from build123d import *

# Parameters (mm, degrees)
SKETCH1_R           = 5.5
SKETCH1_R_2         = 1.5
SKETCH1_R_3         = 4.5
BOSS_EXTRUDE1_DEPTH = 5
SKETCH4_R           = 6.1
CUT_EXTRUDE1_DEPTH  = 3.5
SKETCH5_R           = 1.5
CUT_EXTRUDE2_DEPTH  = 5
SKETCH6_R           = 1.5
CUT_EXTRUDE3_DEPTH  = 10
SKETCH7_R           = 2.9
CUT_EXTRUDE4_DEPTH  = 3.3


with BuildPart() as part:
    # Sketch1 → Boss-Extrude1 (new body)
    with BuildSketch(Plane.XY):
        with BuildLine():
            Line((-58.308676511, 22.996128985), (58.308676511, 22.996128985))
            Line((58.308676511, 22.996128985), (75.629184587, 15))
            Line((75.629184587, 15), (90.85122644, 7.972642053))
            ThreePointArc((90.85122644, 7.972642053), (87.163327852, -21.339018917), (58.308676511, -15))
            Line((58.308676511, -15), (7, -15))
            Line((7, -15), (2.757359313, -19.242640687))
            ThreePointArc((2.757359313, -19.242640687), (0, -20.384776311), (-2.757359313, -19.242640687))
            Line((-2.757359313, -19.242640687), (-7, -15))
            Line((-7, -15), (-58.308676511, -15))
            ThreePointArc((-58.308676511, -15), (-73.76298075, -27.603590324), (-89.217284989, -15))
            ThreePointArc((-89.217284989, -15), (-87.141316573, 1.955509585), (-75.243665272, 14.212949924))
            Line((-75.243665272, 14.212949924), (-58.308676511, 22.996128985))
        make_face()
        with Locations((-74.370815413, -15)):
            Circle(SKETCH1_R, mode=Mode.SUBTRACT)
        with Locations(Location((-74.370815413, -7, 0), (0, 0, 180))):
            Circle(SKETCH1_R_2, mode=Mode.SUBTRACT)
        with Locations((75.629184587, -15)):
            Circle(SKETCH1_R_3, mode=Mode.SUBTRACT)
        with Locations((0, -15.003871015)):
            Circle(SKETCH1_R_2, mode=Mode.SUBTRACT)
        with Locations(Location((-66.370815413, -15, 0), (0, 0, 180))):
            Circle(SKETCH1_R_2, mode=Mode.SUBTRACT)
        with Locations(Location((-74.370815413, -23, 0), (0, 0, 180))):
            Circle(SKETCH1_R_2, mode=Mode.SUBTRACT)
        with Locations(Location((-82.370815413, -15, 0), (0, 0, 180))):
            Circle(SKETCH1_R_2, mode=Mode.SUBTRACT)
        with BuildLine():
            Line((-58.308676511, -4.003871015), (58.308676511, -4.003871015))
            ThreePointArc((58.308676511, -4.003871015), (61.808676511, -0.503871015), (58.308676511, 2.996128985))
            Line((58.308676511, 2.996128985), (-58.308676511, 2.996128985))
            ThreePointArc((-58.308676511, 2.996128985), (-61.808676511, -0.503871015), (-58.308676511, -4.003871015))
        make_face(mode=Mode.SUBTRACT)
    extrude(amount=BOSS_EXTRUDE1_DEPTH)

    # Sketch4 → Cut-Extrude1 (cut)
    with BuildSketch(Plane(origin=(0, 0, 0), x_dir=(-1, 0, 0), z_dir=(0, 0, -1))):
        with Locations((-75.629184587, -15)):
            Circle(SKETCH4_R)
    extrude(amount=-CUT_EXTRUDE1_DEPTH, mode=Mode.SUBTRACT)

    # Sketch5 → Cut-Extrude2 (cut)
    with BuildSketch(Plane(origin=(0, 0, 0), x_dir=(-1, 0, 0), z_dir=(0, 0, -1))):
        with Locations((0, 18.496128985)):
            Circle(SKETCH5_R)
        with Locations((52.5, 18.496128985)):
            Circle(SKETCH5_R)
        with Locations((-52.5, 18.496128985)):
            Circle(SKETCH5_R)
    extrude(amount=-CUT_EXTRUDE2_DEPTH, mode=Mode.SUBTRACT)

    # Sketch6 → Cut-Extrude3 (cut)
    with BuildSketch(Plane(origin=(0, 0, 0), x_dir=(-1, 0, 0), z_dir=(0, 0, -1))):
        with Locations((42.5, -10.5)):
            Circle(SKETCH6_R)
    extrude(amount=-CUT_EXTRUDE3_DEPTH, mode=Mode.SUBTRACT)

    # Sketch7 → Cut-Extrude4 (cut)
    with BuildSketch(Plane(origin=(0, 0, 0), x_dir=(-1, 0, 0), z_dir=(0, 0, -1))):
        with Locations((42.5, -10.5)):
            Circle(SKETCH7_R)
        with Locations((0, -15.003871015)):
            Circle(SKETCH7_R)
        with Locations((0, 18.496128985)):
            Circle(SKETCH7_R)
        with Locations((52.5, 18.496128985)):
            Circle(SKETCH7_R)
        with Locations((-52.5, 18.496128985)):
            Circle(SKETCH7_R)
    extrude(amount=-CUT_EXTRUDE4_DEPTH, mode=Mode.SUBTRACT)


solid = part.part
Geometry: final body of the model. Coordinates: model frame, mm. A direction names the side the tool comes from. Round coordinates to 2 decimals unless told otherwise and drop trailing zeros. Order: outer loops, then holes, each group sorted by start corner. A loop starts at its lowest first (then second) coordinate and runs counter-clockwise, first axis right, second up. Notation, with made-up numbers: (60.25, 62) -> (85.25, 62) arc R17 ccw to (85.25, 75) -> close; hole circle Ø9 at (76, 57.5). An arc over 180 degrees is marked (long way). Put each result on its own line as item: value. Start each with the question number.
Q1. Pull-direction query (X, two-part tool) for faces 1 (the flat face through (-66.895, 18.543, 2.465)), 2 (the cylindrical face through (53.606, 19.51, 4.138)), 3 (the flat face through (-1, 22.996, 2)); classes: +X half, -X half, draft (parallel to the pull), parting line (faces both ways), or undercut.
Q2. Reachability of faces 4 (the flat face through (1, 2.996, 2)), 5 (the flat face through (-32, -15, 2)), 6 (the cylindrical face through (69.994, -17.336, 1.726)) from +Z, -Z, +X, -X, +Y, -Y: full face, straight path, thin tool, end or side. Return the list, or none.
Q3. Line query: probe 1 along Y at (x, z) = (52.5, 1.6); probe 2 along Y at (x, z) = (18.5, 1.85); probe 3 along X at (y, z) = (16, 2.5). Output: solid intervals per line, ascending.
Q4. Section A-A on x = -26.5. Return the cut outline in (y, z).
Q5. First-contact query: pin 1 (1.5 mm diameter, centred on x = 63.5, z = 3.5, fed in from -Y); pin 2 (4.5 mm diameter, centred on x = 0, y = -15, fed in from -Z); pin 3 (14 mm diameter, centred on x = 75.63, y = -15, fed in from -Z); pin 4 (1.5 mm diameter, centred on y = 4.5, z = 1, fed in from +X). Flat tips, straight axial feed; report the tip coordinate or a pass-through.
Q6. Section B-B on z = 2.2. Give the number of separate pieces and of enclosed holes in the cut face, and give its area (3 significant figures).
Ans:
1. face 1: -X half
1. face 2: undercut
1. face 3: draft
2. face 4: +Z, -Z
2. face 5: +Z, -Z, -Y
2. face 6: -Z
3. probe 1: y = -15 to -4, 3 to 15.6, 21.4 to 23
3. probe 2: y = -15 to -4, 3 to 23
3. probe 3: x = -71.8 to -53.98, -51.02 to -1.48, 1.48 to 51.02, 53.98 to 73.46
4. outline: (-15, 0) -> (-4, 0) -> (-4, 5) -> (-15, 5) -> close; (3, 0) -> (23, 0) -> (23, 5) -> (3, 5) -> close
5. pin 1: stops at y = -21.45
5. pin 2: stops at z = 3.3
5. pin 3: stops at z = 0
5. pin 4: stops at x = 93.61
6. separate pieces: 1
6. enclosed holes: 12
6. area: 5,750 mm2
